```python
from build123d import *

# Parameters (mm, degrees)
F1_DEPTH = 7
F2_DEPTH = 6
F3_DEPTH = 15


with BuildPart() as f1:
    # F0 (on Front) → F1 (new body)
    with BuildSketch(Plane.XZ):
        with BuildLine():
            ThreePointArc((-3.477884, 0.719832), (-3.596369, -0.44229), (-3.343322, -1.5827))
            Line((-3.343322, -1.5827), (-3.322458, -1.593981))
            Line((-3.322458, -1.593981), (-3.322458, -2.283465))
            Line((-3.322458, -2.283465), (-2.589551, -2.283465))
            Line((-2.589551, -2.283465), (-2.355576, -2.283465))
            Line((-2.355576, -2.283465), (-2.355576, -2.00205))
            ThreePointArc((-2.355576, -2.00205), (0.063946, 2.771621), (2.483469, -2.00205))
            Line((2.483469, -2.00205), (2.483469, -2.283465))
            Line((2.483469, -2.283465), (2.717444, -2.283465))
            Line((2.717444, -2.283465), (3.450351, -2.283465))
            Line((3.450351, -2.283465), (3.450351, -1.634055))
            ThreePointArc((3.450351, -1.634055), (3.72254, -0.469953), (3.605777, 0.719832))
            ThreePointArc((3.605777, 0.719832), (2.307299, 2.6718), (0.091662, 3.438077))
            ThreePointArc((0.091662, 3.438077), (-2.157419, 2.688675), (-3.477884, 0.719832))
        make_face()
        Polygon((-3.322458, -2.283465), (-3.322458, -1.593981), (-4.089551, -1.943924), (-4.089551, -2.283465), align=None)
        with BuildLine():
            Line((-5.413338, 3.472093), (-3.477884, 0.719832))
            ThreePointArc((-3.477884, 0.719832), (-2.157419, 2.688675), (0.091662, 3.438077))
            Line((0.091662, 3.438077), (-4.408209, 3.472093))
            Line((-4.408209, 3.472093), (-1.413338, 5.938077))
            Line((-1.413338, 5.938077), (-5.413338, 5.938077))
            Line((-5.413338, 5.938077), (-5.413338, 3.472093))
        make_face()
        Polygon((-2.589551, -2.283465), (-3.322458, -2.283465), (-4.089551, -2.283465), (-4.089551, -4.949721), (-3.322458, -4.949721), (-2.589551, -4.949721), align=None)
        with BuildLine():
            Line((4.591534, 3.404061), (0.091662, 3.438077))
            ThreePointArc((0.091662, 3.438077), (2.307299, 2.6718), (3.605777, 0.719832))
            Line((3.605777, 0.719832), (5.587751, 3.472093))
            Line((5.587751, 3.472093), (5.587751, 5.938077))
            Line((5.587751, 5.938077), (1.596662, 5.938077))
            Line((1.596662, 5.938077), (4.591534, 3.404061))
        make_face()
        Polygon((-4.408209, 3.472093), (0.091662, 3.438077), (4.591534, 3.404061), (1.596662, 5.938077), (-1.413338, 5.938077), align=None)
        Polygon((4.217444, -1.943924), (3.450351, -1.634055), (3.450351, -2.283465), (4.217444, -2.283465), align=None)
        Polygon((4.217444, -2.283465), (3.450351, -2.283465), (2.717444, -2.283465), (2.717444, -4.949721), (3.450351, -4.949721), (4.217444, -4.949721), align=None)
    extrude(amount=F1_DEPTH)

    # F0 (on Front) → F2 (cut)
    with BuildSketch(Plane.XZ):
        Polygon((-4.408209, 3.472093), (0.091662, 3.438077), (4.591534, 3.404061), (1.596662, 5.938077), (-1.413338, 5.938077), align=None)
    extrude(amount=F2_DEPTH, mode=Mode.SUBTRACT)

    # F0 (on Front) → F3 (join)
    with BuildSketch(Plane.XZ):
        Polygon((4.217444, -2.283465), (3.450351, -2.283465), (2.717444, -2.283465), (2.717444, -4.949721), (3.450351, -4.949721), (4.217444, -4.949721), align=None)
        Polygon((-2.589551, -2.283465), (-3.322458, -2.283465), (-4.089551, -2.283465), (-4.089551, -4.949721), (-3.322458, -4.949721), (-2.589551, -4.949721), align=None)
    extrude(amount=-F3_DEPTH)


solid = f1.part
```
Verification items for the finished model (mm, model axes). A direction names the side the tool comes from. Round coordinates to 2 decimals unless told otherwise and drop trailing zeros. Write each loop counter-clockwise with the first axis right and the second up, starting at its lowest first coordinate (ties: lowest second). Pieces come first, ordered by that corner, then holes. Notation, with made-up numbers: (-17, 63.25) -> (-2, 63.25) arc R26 ccw to (-2, 95.25) -> close; hole circle Ø5 at (70.25, 64). An arc over 180 degrees is marked (long way). Write each question's results on one line, items separated by ' | '. Start each with the question number.
1. Depth check by flat-ended pin: P1, Ø3, axis at y = 6, z = -1.5, coming from the +X side; P2, Ø0.8, axis at x = 3.5, y = 5, coming from the +Z side; P3, Ø2, axis at y = 7, z = -4, coming from the -X side; P4, Ø1.5, axis at x = 0, z = -2.5, coming from the +Y side. Enter the tip coordinate at first touch or a pass-through.
2. Cross-section at B-B (y = 9.75). Enter the section's corners in (x, z).
3. Cross-section at C-C (x = 4). Enter the section's corners in (y, z).
4. Set-up check for faces 5 (the flat face through (4.6, -3.5, 2.1)), 6 (the flat face through (0, 0, 3)), 7 (the flat face through (2.717, 4, -4)), 8 (the flat face through (3.12, -2.96, 4.65)): record each of +Z, -Z, +X, -X, +Y, -Y from which the full face is reachable in a straight line by a thin tool's end or side.
5. Cross-section at A-A (z = -2.75). Enter the section's corners in (x, y), then the cut area to 3 significant figures.
6. Material ranges on probe 1 along X at (y, z) = (-5.5, -0.25); probe 2 along X at (y, z) = (-3.5, -2.5); probe 3 along Y at (x, z) = (0.25, 3), recorded low to high. Write a range as from..to.
7. Draft check along X on faces 1 (the flat face through (-4.09, 4, -3)), 2 (the flat face through (-2.89, -2.96, 4.72)), 3 (the cylindrical face through (-0.03, -3.45, 2.77)), 4 (the cylindrical face through (3.72, -3.45, -0.49)). Enter one of: +X half, -X half, draft (parallel to the pull), parting line (faces both ways), or undercut.
Solutions:
1) P1: stops at x = 4.22 | P2: stops at z = -2.28 | P3: stops at x = -4.09 | P4: passes through
2) outline: (-4.09, -4.95) -> (-2.59, -4.95) -> (-2.59, -2.28) -> (-4.09, -2.28) -> close; (2.72, -4.95) -> (4.22, -4.95) -> (4.22, -2.28) -> (2.72, -2.28) -> close
3) outline: (-7, -4.95) -> (15, -4.95) -> (15, -2.28) -> (0, -2.28) -> (0, -1.86) -> (-7, -1.86) -> close; (-7, 1.27) -> (0, 1.27) -> (0, 3.41) -> (-6, 3.41) -> (-6, 3.9) -> (0, 3.9) -> (0, 5.94) -> (-7, 5.94) -> close
4) face 5: +X, +Y, -Y | face 6: +Z, +X, -X, +Y | face 7: -Z, +Y, -Y | face 8: +Y
5) outline: (-4.09, -7) -> (-2.59, -7) -> (-2.59, 15) -> (-4.09, 15) -> close; (2.72, -7) -> (4.22, -7) -> (4.22, 15) -> (2.72, 15) -> close | area: 66.0 mm2
6) probe 1: x = -3.6..-2.94, 3.06..3.73 | probe 2: x = -4.09..-2.59, 2.72..4.22 | probe 3: y = -7..0
7) face 1: -X half | face 2: undercut | face 3: undercut | face 4: +X half
